Autodesk Fusion 360 part; units mm, degrees
sketch "Sketch1" plane through (0, 0, 0) normal (0, 1, 0) x (1, 0, 0)
  circle A0 centre (0, 0) radius 26
  line L0 (0, 0) -> (22.5167, 13)
  line L1 (0, 0) -> (26, 0) construction
  line L2 (0, 0) -> (-22.5167, 13)
  line L3 (0, 0) -> (26, 0) construction
  line L4 (0, 0) -> (0, -26)
  circle A1 centre (0, 0) radius 23.5
  circle A2 centre (0, 0) radius 28.5
  line L5 (-22.5167, 13) -> (-22.5167, 16)
  line L6 (-22.5167, 13) -> (-22.5167, 10)
  line L7 (-24.1667, 10) -> (-24.1667, 16)
  line L8 (-20.8667, 10) -> (-20.8667, 16)
  line L9 (0, -26) -> (0, -23)
  line L10 (0, -26) -> (0, -29)
  line L11 (0, -26) -> (0, -23)
  line L12 (0, -29) -> (-1.65, -29)
  line L13 (-1.65, -29) -> (-1.65, -23)
  line L14 (1.65, -23) -> (1.65, -29)
  line L15 (24.1667, 10) -> (24.1667, 16)
  line L16 (20.8667, 10) -> (20.8667, 16)
  arc A3 (-1.65, -29) -> (1.65, -29) centre (0, -29) ccw
  arc A4 (1.65, -23) -> (-1.65, -23) centre (0, -23) ccw
  arc A5 (20.8667, 10) -> (24.1667, 10) centre (22.5167, 10) ccw
  arc A6 (24.1667, 16) -> (20.8667, 16) centre (22.5167, 16) ccw
  arc A7 (-24.1667, 10) -> (-20.8667, 10) centre (-22.5167, 10) ccw
  arc A8 (-20.8667, 16) -> (-24.1667, 16) centre (-22.5167, 16) ccw
  line L17 (-25.6667, 10) -> (-25.6667, 16)
  arc A9 (-19.3667, 16) -> (-25.6667, 16) centre (-22.5167, 16) ccw
  line L18 (-19.3667, 10) -> (-19.3667, 16)
  arc A10 (-25.6667, 10) -> (-19.3667, 10) centre (-22.5167, 10) ccw
  line L19 (-3.15, -29) -> (-3.15, -23)
  arc A11 (3.15, -23) -> (-3.15, -23) centre (0, -23) ccw
  line L20 (3.15, -23) -> (3.15, -29)
  arc A12 (-3.15, -29) -> (3.15, -29) centre (0, -29) ccw
  line L21 (19.3667, 10) -> (19.3667, 16)
  arc A13 (25.6667, 16) -> (19.3667, 16) centre (22.5167, 16) ccw
  line L22 (25.6667, 10) -> (25.6667, 16)
  arc A14 (19.3667, 10) -> (25.6667, 10) centre (22.5167, 10) ccw
  dimension "d1" = 52
  dimension "d2" = 30
  dimension "d3" = 150
  dimension "d7" = 47
  dimension "d8" = 57
  dimension "d9" = 3
  dimension "d11" = 3.3
  dimension "d12" = 3
  dimension "d13" = 3
  dimension "d14" = 3.3
  dimension "d15" = 3.3
  dimension "d23" = 1.5
  dimension "d24" = 1.5
  dimension "d25" = 1.5
extrude "Extrude2" add sketch "Sketch1" along normal blind 3 contours A0 A1 L20 A14 | A0 A2 L20 L22 A14 | A0 A1 A5 A14 | A0 A2 L15 A5 L22 A14 | A0 A2 L14 L20 | A0 A1 L14 L20 | L0 A1 L16 A5 L21 A14 | L4 A1 L14 A4 A11 L20 | A2 L13 L14 A3 L19 L20 A12 | A2 L15 A6 A13 L22 | A0 L0 A1 L16 L21 A13 | A0 A2 L16 A6 A13 | L0 A1 L16 | L0 A1 L21 | A0 A2 L13 L19 | A0 A1 L13 L19 | L4 A1 L13 A4 L19 A11 | A0 A1 A9 L18 L21 A13 | A0 A2 A9 A13 | A0 A2 L17 A10 L19 | A0 A1 A10 L19 | A0 L2 A1 L8 A9 L18 | A0 A2 L8 A8 A9 | L2 A1 L8 A7 L18 A10 | L2 A1 L18 | A2 L7 A8 L17 A9 | A0 A2 L7 A7 L17 A10 | A0 A1 A7 A10 | L2 A1 L8
sketch "Sketch2" plane through (0, 3, 0) normal (0, 1, 0) x (-1, 0, 0)
  arc A0 (-20.8667, -10) -> (-24.1667, -10) centre (-22.5167, -10) ccw
  line L0 (-20.8667, -10) -> (-20.8667, -16)
  arc A1 (-24.1667, -16) -> (-20.8667, -16) centre (-22.5167, -16) ccw
  line L1 (-24.1667, -16) -> (-24.1667, -10)
  arc A2 (24.1667, -10) -> (20.8667, -10) centre (22.5167, -10) ccw
  line L2 (24.1667, -10) -> (24.1667, -16)
  arc A3 (20.8667, -16) -> (24.1667, -16) centre (22.5167, -16) ccw
  line L3 (20.8667, -16) -> (20.8667, -10)
  arc A4 (1.65, 29) -> (-1.65, 29) centre (0, 29) ccw
  line L4 (1.65, 29) -> (1.65, 23)
  arc A5 (-1.65, 23) -> (1.65, 23) centre (0, 23) ccw
  line L5 (-1.65, 23) -> (-1.65, 29)
  arc A6 (-19.3667, -13.311) -> (19.3667, -13.311) centre (0, 0) ccw
  line L6 (-19.3667, -13.311) -> (-19.3667, -10)
  arc A7 (-19.3667, -10) -> (-22.4794, -6.8502) centre (-22.5167, -10) ccw
  arc A8 (-3.15, 23.2879) -> (-22.4794, -6.8502) centre (0, 0) ccw
  line L7 (-3.15, 23.2879) -> (-3.15, 23)
  arc A9 (-3.15, 23) -> (3.15, 23) centre (0, 23) ccw
  line L8 (3.15, 23) -> (3.15, 23.2879)
  arc A10 (22.4794, -6.8502) -> (3.15, 23.2879) centre (0, 0) ccw
  arc A11 (22.4794, -6.8502) -> (19.3667, -10) centre (22.5167, -10) ccw
  line L9 (19.3667, -10) -> (19.3667, -13.311)
  arc A12 (3.15, 29) -> (-3.15, 29) centre (0, 29) ccw
  line L10 (-3.15, 29) -> (-3.15, 28.3254)
  arc A13 (-3.15, 28.3254) -> (-25.6667, -12.3884) centre (0, 0) ccw
  line L11 (-25.6667, -12.3884) -> (-25.6667, -16)
  arc A14 (-25.6667, -16) -> (-21.3196, -18.9137) centre (-22.5167, -16) ccw
  arc A15 (-21.3196, -18.9137) -> (21.3196, -18.9137) centre (0, 0) ccw
  arc A16 (21.3196, -18.9137) -> (25.6667, -16) centre (22.5167, -16) ccw
  line L12 (25.6667, -16) -> (25.6667, -12.3884)
  arc A17 (25.6667, -12.3884) -> (3.15, 28.3254) centre (0, 0) ccw
  line L13 (3.15, 28.3254) -> (3.15, 29)
  circle A18 centre (0, 0) radius 23.75
  circle A19 centre (0, 0) radius 30
  circle A20 centre (0, 0) radius 25 construction
  circle A21 centre (0, 0) radius 27.5 construction
  line L14 (0, 0) -> (0, -35)
  line L15 (0, 0) -> (-30.3109, 17.5)
  line L16 (0, 0) -> (35, 0) construction
  line L17 (0, 0) -> (30.3109, 17.5)
  line L18 (0, 0) -> (35, 0) construction
  circle A22 centre (30.3109, 17.5) radius 1.65
  circle A23 centre (-30.3109, 17.5) radius 1.65
  circle A24 centre (0, -35) radius 1.65
  circle A25 centre (0, -35) radius 3
  circle A26 centre (30.3109, 17.5) radius 3
  circle A27 centre (-30.3109, 17.5) radius 3
  line L19 (-30.3109, 17.5) -> (-31.8109, 14.9019)
  line L20 (-31.8109, 14.9019) -> (-27.3505, 12.3267)
  line L21 (-30.3109, 17.5) -> (-28.8109, 20.0981)
  line L22 (-28.8109, 20.0981) -> (-24.3505, 17.5229)
  line L23 (31.8109, 14.9019) -> (27.3505, 12.3267)
  line L24 (28.8109, 20.0981) -> (24.3505, 17.5229)
  line L25 (3, -35) -> (3, -29.8496)
  line L26 (0, -35) -> (3, -35)
  line L27 (0, -35) -> (-3, -35)
  line L28 (-3, -35) -> (-3, -29.8496)
  dimension "d28" = 47.5
  dimension "d29" = 60
  dimension "d32" = 50
  dimension "d33" = 55
  dimension "d39" = 35
  dimension "d40" = 150
  dimension "d41" = 35
  dimension "d42" = 35
  dimension "d43" = 30
  dimension "d44" = 3.3
  dimension "d45" = 3.3
  dimension "d46" = 3.3
  dimension "d47" = 6
  dimension "d48" = 6
  dimension "d49" = 6
extrude "Extrude3" add sketch "Sketch2" against normal blind 3 contours A12 L10 A13 A19 L15 | A13 L11 A19 L15 | A14 A15 A19 L14 | A15 A16 A19 L14 | A19 L15 A27 L22 | A19 L15 A27 L20 | A19 L14 A25 L28 | A19 L14 A25 L25 | L15 A23 A27 L19 | L15 A23 A27 L21 | L14 A24 A25 L26 | L14 A24 A25 L27 | L12 A17 A19 L17 | A12 A17 L13 A19 L17 | A23 A27 L19 L21 | A24 A25 L26 L27 | A19 L17 A26 L23 | A19 L17 A26 L24 | A26
fillet "Fillet1" radius 2 6 edges at (-24.3505, 1.5, 17.5229) (-27.3505, 1.5, 12.3267) (-3, 1.5, -29.8496) (3, 1.5, -29.8496) (27.3505, 1.5, 12.3267) (24.3505, 1.5, 17.5229)
equation "d1 = ( 26 * 2 ) * 1 mm"
equation "d8 = 52 mm + 5 mm"
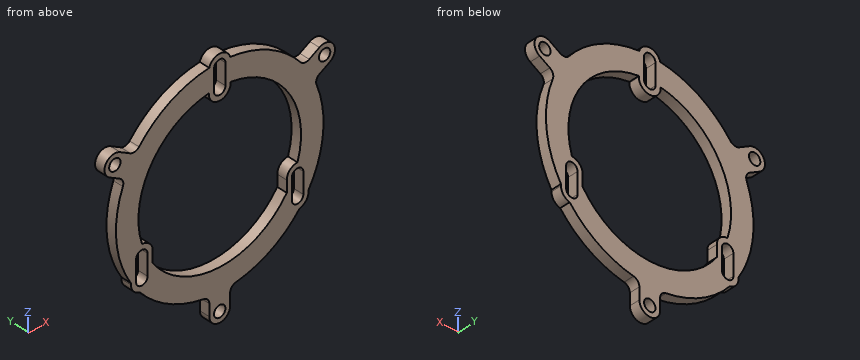
CAD build for the part. Positions are in the model's coordinates, mm. Round coordinates to 2 decimals unless told otherwise and drop trailing zeros. Loops run counter-clockwise (first coordinate to the right, second up) from the corner with the lowest first, then second, coordinate; pieces in that order, holes last. Notation, with made-up numbers: M -19.5,77.25 L -14.5,77.25 A8 cw -14.5,85.25 Z; hole C 58.25,55 d9. An arc over 180 degrees is marked long. Return JSON: item names as keys, results as strings. Group by question number.
(1) Saw through at D-D, the plane y = 2.2. Give the number of separate pieces and of enclosed holes in the cut face, and give its area (3 significant figures).
(2) Saw through at A-A, the plane z = 0. List the corners of the cut face in (x, y), and give its area (3 significant figures).
(3) Saw through at C-C, the plane z = -26.5. List the corners of the cut face in (x, y).
(4) Wall check: probe 1 along X at (y, z) = (0.8, 17.5); probe 2 along X at (y, z) = (2.3, -35); probe 3 along X at (y, z) = (1.05, -12). Give the ranges that are in metal, low to high. Write a range as [from, to].
(5) Saw through at B-B, the plane x = 15.5. List the corners of the cut face in (y, z).
(6) Drop flat-ended pins along their axis: P1, Ø2, axis at x = -30.31, z = 17.5, coming from the -Y side; P2, Ø1, axis at x = -2, y = 2.5, coming from the +Z side; P3, Ø0.5, axis at y = 1, z = -16, coming from the +X side; P4, Ø0.9, axis at y = 2, z = -11.5, coming from the -X side. Give the stop position or say it passes through.
Answer list:
{
 "1": {"separate pieces": "1", "enclosed holes": "7", "area": "1,170 mm2"},
 "2": {"outline": "M -30,0 L -23.5,0 L -23.5,3 L -30,3 Z; M 23.5,0 L 30,0 L 30,3 L 23.5,3 Z", "area": "39.0 mm2"},
 "3": {"outline": "M -14.06,0 L 14.06,0 L 14.06,3 L -14.06,3 Z"},
 "4": {"probe 1": "[-33.31, -31.96], [-28.66, -15.68], [15.68, 28.66], [31.96, 33.31]", "probe 2": "[-3, -1.65], [1.65, 3]", "probe 3": "[-27.5, -24.17], [-20.87, -19.37], [19.37, 20.87], [24.17, 27.5]"},
 "5": {"outline": "M 0,-25.69 L 3,-25.69 L 3,-17.66 L 0,-17.66 Z; M 0,17.66 L 3,17.66 L 3,25.69 L 0,25.69 Z"},
 "6": {"P1": "through", "P2": "z = 31.77", "P3": "x = 25.67", "P4": "x = -27.89"}
}
